For this review, take the finished solid that the model builds, in its own axes (mm). A direction names the side the tool comes from. Round coordinates to 2 decimals unless told otherwise and drop trailing zeros. Loops run counter-clockwise (first coordinate to the right, second up) from the corner with the lowest first, then second, coordinate; pieces in that order, holes last.
1) Tool access review of faces 5 (the flat face through (6, 0, -6)), 6 (the flat face through (0.635, 1, -6)): name each direction out of +Z, -Z, +X, -X, +Y, -Y from which nothing blocks a thin tool from reaching the whole face with its end or side.
2) Take a section at A-A (y = 0.9). State the section outline as (x, z) points (3 decimals).
3) Wall thickness on L1, parallel to X at y = 0.55, z = -1.5 (3 decimals); L2, parallel to X at y = 1.35, z = -8.5 (3 decimals); L3, parallel to Z at x = 1, y = 1.2 (3 decimals): over which ranges is each line inside the solid? List them lowest first.
4) Mouldability with a two-part tool opening along X and no side actions: class faces 1 (the flat face through (5, 1.905, -9)), 2 (the flat face through (12.065, 1, -6)), 3 (the flat face through (6.24, 2.543, -4.8)), 4 (the flat face through (12.7, 1, -6)) as pulls with the +X half, pulls with the -X half, needs draft (parallel to the pull), parting line crosses it, or undercut.
5) Take a section at B-B (x = 10.5). State the section outline as (y, z) points (3 decimals), then the cut area to 3 significant figures.
6) Insertion check: pin 1 (1 mm diameter, centred on x = 10, z = -7.5, fed in from -Y) (3 decimals). The pin has a flat end and moves straight along its axis. Give the tip position at first contact, or say it passes through.
7) Take a section at D-D (x = 7.5). State the section outline as (y, z) points (3 decimals).
8) Take a section at C-C (z = -1.25). State the section outline as (x, y) points (3 decimals).
```python
from build123d import *

# Parameters (mm, degrees)
SKETCH1_W           = 12.7
SKETCH1_H           = 12.7
BOSS_EXTRUDE1_DEPTH = 2.54
FILLET1_R           = 0.635
SHELL1_START        = 0.635
SHELL1_OUTLINE_W    = 1.905
SHELL1_OUTLINE_H    = 11.43
SHELL1_DEPTH        = 11.43
SKETCH2_R           = 2.54
BOSS_EXTRUDE2_DEPTH = 1.905
BOSS_EXTRUDE3_DEPTH = 0.00254


# Read off the part's stored shape, not the designer's step: Shell1
with BuildPart() as part:
    # Sketch1 → Boss-Extrude1 (new body)
    with BuildSketch(Plane(origin=(0, 0, 0), x_dir=(1, 0, 0), z_dir=(0, 1, 0))):
        with Locations((6.35, 6.35)):
            Rectangle(SKETCH1_W, SKETCH1_H)
    extrude(amount=BOSS_EXTRUDE1_DEPTH)

    # Fillet1
    fillet1_edges = [part.edges().sort_by_distance(p)[0] for p in [
        (0, 1.27, -12.7),
        (12.7, 1.27, -12.7),
        (12.7, 1.27, 0),
        (0, 1.27, 0),
    ]]
    fillet(fillet1_edges, radius=FILLET1_R)

    # Shell1 outline → Shell1 (cut)
    with BuildSketch(Plane.YZ.offset(SHELL1_START)):
        with Locations((0.9525, -6.35)):
            Rectangle(SHELL1_OUTLINE_W, SHELL1_OUTLINE_H)
    extrude(amount=SHELL1_DEPTH, mode=Mode.SUBTRACT)

    # Sketch2 → Boss-Extrude2 (add)
    with BuildSketch(Plane(origin=(0, 1.905, 0), x_dir=(-1, 0, 0), z_dir=(0, -1, 0))):
        with Locations(Location((-6.35, 6.35, 0), (0, 0, 270))):
            Circle(SKETCH2_R)
    extrude(amount=BOSS_EXTRUDE2_DEPTH)

    # Sketch3 → Boss-Extrude3 (add)
    with BuildSketch(Plane(origin=(0, 2.54, 0), x_dir=(1, 0, 0), z_dir=(0, 1, 0))):
        with BuildLine():
            Line((5.853397436, 10.234897436), (5.283525641, 10.234897436))
            add(Edge.make_bspline(
                [(5.283525641, 10.234897436), (5.284353116, 10.268014374), (5.285977943, 10.333042737), (5.299594671, 10.4283349), (5.322170454, 10.519147471), (5.352113733, 10.606188577), (5.393180841, 10.687937495), (5.441181448, 10.76617845), (5.499755897, 10.839002803), (5.544084465, 10.883394842), (5.566553486, 10.905896034)],
                knots=[0, 0, 0, 0, 1.059318936, 2.080076833, 3.072188589, 4.050544838, 5.018331365, 5.993389509, 6.98290034, 8, 8, 8, 8], degree=3))
            add(Edge.make_bspline(
                [(5.566553486, 10.905896034), (5.590433678, 10.927308972), (5.638116529, 10.970065325), (5.718689808, 11.022828021), (5.803504931, 11.06921666), (5.894268619, 11.106972474), (5.990827059, 11.135076524), (6.092587635, 11.156569797), (6.200177048, 11.168294409), (6.273779262, 11.170162374), (6.311330128, 11.171115385)],
                knots=[0, 0, 0, 0, 0.948883556, 1.894686314, 2.844483856, 3.810176973, 4.799693044, 5.819515431, 6.887545887, 8, 8, 8, 8], degree=3))
            add(Edge.make_bspline(
                [(6.311330128, 11.171115385), (6.359120103, 11.169889945), (6.451588454, 11.167518855), (6.584514069, 11.146011833), (6.706975805, 11.112324433), (6.817814436, 11.062735489), (6.918012523, 11.000478686), (7.007887309, 10.926220415), (7.086994083, 10.839200529), (7.15395512, 10.741225072), (7.209386328, 10.636664029), (7.249233878, 10.527377386), (7.273840561, 10.415142851), (7.276663402, 10.339114174), (7.278076923, 10.301043269)],
                knots=[0, 0, 0, 0, 1.182572727, 2.288148342, 3.325075675, 4.319152577, 5.283495877, 6.237943501, 7.196683647, 8.185423483, 9.169287591, 10.119220246, 11.058210795, 12, 12, 12, 12], degree=3))
            add(Edge.make_bspline(
                [(7.278076923, 10.301043269), (7.277544158, 10.280036013), (7.276486473, 10.238330852), (7.269296582, 10.176000543), (7.257269416, 10.114301607), (7.239843882, 10.052905415), (7.217550967, 9.991355497), (7.188970888, 9.929663399), (7.156358228, 9.866252998), (7.13002819, 9.825307022), (7.116528446, 9.804313502)],
                knots=[0, 0, 0, 0, 0.951041345, 1.888077725, 2.83683973, 3.794061122, 4.774862461, 5.797242242, 6.870618167, 8, 8, 8, 8], degree=3))
            add(Edge.make_bspline(
                [(7.116528446, 9.804313502), (7.111705931, 9.797489865), (7.101130556, 9.782526193), (7.082517064, 9.75891757), (7.059541503, 9.732239397), (7.032124964, 9.702588546), (7.000954688, 9.669311823), (6.965245373, 9.633134756), (6.925180303, 9.593688673), (6.896720873, 9.566610908), (6.881837941, 9.552450521)],
                knots=[0, 0, 0, 0, 0.581581733, 1.275360758, 2.091728324, 3.031843472, 4.086285973, 5.265534873, 6.570004409, 8, 8, 8, 8], degree=3))
            add(Edge.make_bspline(
                [(6.881837941, 9.552450521), (6.867823063, 9.538905104), (6.840980246, 9.512961451), (6.802850531, 9.475403757), (6.768477971, 9.441288703), (6.738583417, 9.410113726), (6.712767428, 9.382030868), (6.691628482, 9.356598526), (6.673181109, 9.335190758), (6.655268183, 9.309193967), (6.636134141, 9.27630329), (6.617692661, 9.232315394), (6.598752582, 9.183656029), (6.583064675, 9.127819109), (6.568525728, 9.063850691), (6.558444173, 8.98913819), (6.550158775, 8.903425503), (6.54703617, 8.842461817), (6.545384615, 8.810217949)],
                knots=[0, 0, 0, 0, 1.102030995, 2.110729467, 3.026154581, 3.840042361, 4.552846469, 5.182140586, 5.710117496, 6.149081041, 6.965348744, 7.856273241, 8.842571802, 9.916136751, 11.13180819, 12.549025941, 14.174769928, 16, 16, 16, 16], degree=3))
            Line((6.545384615, 8.810217949), (5.977420873, 8.810217949))
            Line((5.977420873, 8.810217949), (5.975512821, 8.906256611))
            add(Edge.make_bspline(
                [(5.975512821, 8.906256611), (5.976741281, 8.952959078), (5.97915227, 9.04461782), (5.997923184, 9.17890025), (6.028889585, 9.306674594), (6.073183888, 9.428411842), (6.13183631, 9.545115416), (6.206199488, 9.657101789), (6.295918801, 9.765710318), (6.365304252, 9.831931248), (6.401008614, 9.866007212)],
                knots=[0, 0, 0, 0, 1.033439605, 2.028239196, 2.994517618, 3.938676781, 4.889343937, 5.878493955, 6.908315515, 8, 8, 8, 8], degree=3))
            add(Edge.make_bspline(
                [(6.401008614, 9.866007212), (6.418203829, 9.881882491), (6.451045739, 9.912203398), (6.497521564, 9.955831899), (6.538207001, 9.996143513), (6.574021852, 10.032027952), (6.60360938, 10.064736512), (6.629111702, 10.092412527), (6.647857862, 10.117289473), (6.667224093, 10.144496763), (6.683688858, 10.178654576), (6.697823373, 10.221420023), (6.707139354, 10.267146407), (6.707845528, 10.298877478), (6.708205128, 10.315035657)],
                knots=[0, 0, 0, 0, 1.496681724, 2.858579316, 4.076169266, 5.159545538, 6.0998563, 6.897021917, 7.564130093, 8.090631505, 9.030453413, 9.97369198, 10.968158133, 12, 12, 12, 12], degree=3))
            add(Edge.make_bspline(
                [(6.708205128, 10.315035657), (6.706888341, 10.337037285), (6.704281107, 10.380600413), (6.682492098, 10.442939177), (6.645885475, 10.499075222), (6.596763053, 10.549162809), (6.535851582, 10.591103493), (6.464068799, 10.621322106), (6.382800734, 10.639196819), (6.325417451, 10.641004203), (6.295429687, 10.641948718)],
                knots=[0, 0, 0, 0, 0.89686541, 1.775789589, 2.659646804, 3.614799273, 4.623469819, 5.659165238, 6.776709961, 8, 8, 8, 8], degree=3))
            add(Edge.make_bspline(
                [(6.295429687, 10.641948718), (6.264541595, 10.640790498), (6.204905733, 10.638554313), (6.119938634, 10.616043899), (6.04348174, 10.580249645), (5.977164014, 10.530348621), (5.922544381, 10.469360961), (5.883350326, 10.398410103), (5.85768066, 10.319511854), (5.854856732, 10.263725594), (5.853397436, 10.234897436)],
                knots=[0, 0, 0, 0, 1.100648509, 2.125029966, 3.113637804, 4.097598811, 5.068105762, 6.013525516, 6.973467682, 8, 8, 8, 8], degree=3))
        make_face()
        with BuildLine():
            add(Edge.make_bspline(
                [(6.275713141, 8.525282051), (6.299179014, 8.524134389), (6.345232632, 8.521882012), (6.411126908, 8.501852518), (6.471995891, 8.470197401), (6.524870844, 8.425537098), (6.570385609, 8.37347305), (6.603443799, 8.313958987), (6.623341923, 8.248804438), (6.62562935, 8.203595823), (6.626794872, 8.180560497)],
                knots=[0, 0, 0, 0, 1.02832881, 2.018176019, 2.996839149, 4.02200224, 5.038888337, 6.018215493, 6.990213417, 8, 8, 8, 8], degree=3))
            add(Edge.make_bspline(
                [(6.626794872, 8.180560497), (6.625666727, 8.157301936), (6.623462536, 8.11185888), (6.603201866, 8.046543983), (6.571118549, 7.986459509), (6.526395492, 7.933679904), (6.473728692, 7.88919342), (6.413890891, 7.85658064), (6.348398585, 7.836741414), (6.302775693, 7.834458232), (6.279529247, 7.833294872)],
                knots=[0, 0, 0, 0, 1.020984004, 1.994819617, 2.979715589, 3.999633825, 5.019552061, 5.996242457, 6.979015996, 8, 8, 8, 8], degree=3))
            add(Edge.make_bspline(
                [(6.279529247, 7.833294872), (6.25649052, 7.834451139), (6.211275231, 7.836720402), (6.14626792, 7.856720874), (6.086621496, 7.889203344), (6.03394775, 7.933503713), (5.989781247, 7.986503553), (5.958510337, 8.046704841), (5.938103298, 8.111841812), (5.935923402, 8.157296158), (5.934807692, 8.180560497)],
                knots=[0, 0, 0, 0, 1.015319757, 1.992643789, 2.97283283, 3.99640456, 5.014008891, 5.998034653, 6.975358685, 8, 8, 8, 8], degree=3))
            add(Edge.make_bspline(
                [(5.934807692, 8.180560497), (5.93601664, 8.203587923), (5.938386138, 8.248720962), (5.957566002, 8.313737697), (5.989195997, 8.373406988), (6.033493364, 8.425503873), (6.085003898, 8.469937879), (6.144023925, 8.50185823), (6.208070436, 8.521877137), (6.252880831, 8.524132747), (6.275713141, 8.525282051)],
                knots=[0, 0, 0, 0, 1.024777805, 2.008532629, 2.993375778, 4.013176149, 5.039042267, 6.007247738, 6.984629846, 8, 8, 8, 8], degree=3))
        make_face()
        Polygon((5.288410256, 2.732128205), (6.749342748, 6.558410256), (7.181198718, 6.558410256), (5.720266226, 2.732128205), align=None)
    extrude(amount=BOSS_EXTRUDE3_DEPTH)


solid = part.part
```
Response:
1. face 5: +Z, -Z, +X, -X, -Y
1. face 6: -Y
2. outline: (0, -12.065) arc R0.635 ccw to (0.635, -12.7) - (12.065, -12.7) arc R0.635 ccw to (12.7, -12.065) - (12.7, -0.635) arc R0.635 ccw to (12.065, 0) - (0.635, 0) arc R0.635 ccw to (0, -0.635) - close; circle Ø5.08 at (6.35, -6.35); hole (0.635, -12.065) - (12.065, -12.065) - (12.065, -0.635) - (0.635, -0.635) - close
3. L1: x = 0 to 0.635, 12.065 to 12.7
3. L2: x = 0 to 0.635, 4.998 to 7.702, 12.065 to 12.7
3. L3: z = -12.7 to -12.065, -0.635 to 0
4. face 1: undercut
4. face 2: undercut
4. face 3: needs draft
4. face 4: pulls with the +X half
5. outline: (0, -12.7) - (2.54, -12.7) - (2.54, 0) - (0, 0) - (0, -0.635) - (1.905, -0.635) - (1.905, -12.065) - (0, -12.065) - close
5. area: 10.5 mm2
6. pin 1: stops at y = 1.905
7. outline: (0, -12.7) - (2.54, -12.7) - (2.54, 0) - (0, 0) - (0, -0.635) - (1.905, -0.635) - (1.905, -4.085) - (0, -4.085) - (0, -8.615) - (1.905, -8.615) - (1.905, -12.065) - (0, -12.065) - close
8. outline: (0, 0) - (0.635, 0) - (0.635, 1.905) - (12.065, 1.905) - (12.065, 0) - (12.7, 0) - (12.7, 2.54) - (0, 2.54) - close
